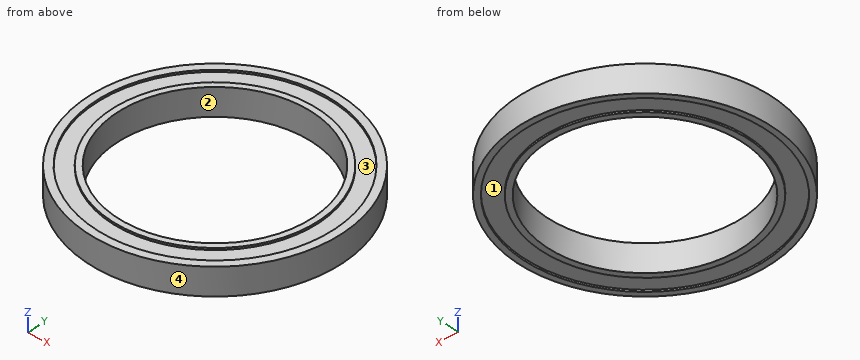
from build123d import *

# Parameters (mm, degrees)
SKETCH010_R     = 32.5
SKETCH010_R_2   = 25
PAD007_DEPTH    = 7
SKETCH011_R     = 30.5
SKETCH011_R_2   = 26.5
POCKET004_DEPTH = 0.5
SKETCH012_R     = 31
SKETCH012_R_2   = 26.5
POCKET005_DEPTH = 0.5


with BuildPart() as part:
    # Sketch010 → Pad007 (new body)
    with BuildSketch(Plane.XY):
        Circle(SKETCH010_R)
        Circle(SKETCH010_R_2, mode=Mode.SUBTRACT)
    extrude(amount=PAD007_DEPTH)

    # Sketch011 → Pocket004 (cut)
    with BuildSketch(Plane.XY.offset(7)):
        Circle(SKETCH011_R)
        Circle(SKETCH011_R_2, mode=Mode.SUBTRACT)
    extrude(amount=-POCKET004_DEPTH, mode=Mode.SUBTRACT)

    # Sketch012 → Pocket005 (cut)
    with BuildSketch(Plane.XY):
        Circle(SKETCH012_R)
        Circle(SKETCH012_R_2, mode=Mode.SUBTRACT)
    extrude(amount=POCKET005_DEPTH, mode=Mode.SUBTRACT)


solid = part.part
Design review of the part built by this model. Coordinates are the model's own, in mm. Face numbers are marked on the shaded views. A direction names the side the tool comes from. Round coordinates to 2 decimals unless told otherwise and drop trailing zeros. Order: outer loops, then holes, each group sorted by start corner. A loop starts at its lowest first (then second) coordinate and runs counter-clockwise, first axis right, second up.
1) Draft analysis for pull direction Y (two halves, no side actions). For the marked faces 3 and 4, state which applies: released by +Y, released by -Y, zero draft, split by the parting line, or undercut.
The answers:
face 3: undercut
face 4: split by the parting line
2) Consider section A-A (y = 0). State the section outline as (x, z) points.
The answers:
outline: (-32.5, 0) - (-31, 0) - (-31, 0.5) - (-26.5, 0.5) - (-26.5, 0) - (-25, 0) - (-25, 7) - (-26.5, 7) - (-26.5, 6.5) - (-30.5, 6.5) - (-30.5, 7) - (-32.5, 7) - close; (25, 0) - (26.5, 0) - (26.5, 0.5) - (31, 0.5) - (31, 0) - (32.5, 0) - (32.5, 7) - (30.5, 7) - (30.5, 6.5) - (26.5, 6.5) - (26.5, 7) - (25, 7) - close
3) Clearance check with flat-ended pins moving along their axes: pin 1 Ø2 at (y, z) = (24, 3) entering from +X; pin 2 Ø2 at (y, z) = (-25, 3.5) entering from -X; pin 3 Ø1.5 at (x, y) = (-21, -24.5) entering from -Z; pin 4 Ø2 at (x, y) = (-20, -11) entering from +Z. State where each tip first meets the part, or that it passes through.
The answers:
pin 1: stops at x = 22.96
pin 2: stops at x = -21.91
pin 3: stops at z = 0
pin 4: passes through
4) Consider section C-C (z = 2.25). State the section outline as (x, y) points.
The answers:
outline: circle Ø65 at (0, 0); hole circle Ø50 at (0, 0)
5) For L1, parallel to Y at x = 0, z = 6.85; L2, parallel to Y at x = 0, z = 0.45; L3, parallel to Y at x = 0, z = 3, list the stretches that pass through material, from the lowest coordinate up.
The answers:
L1: y = -32.5 to -30.5, -26.5 to -25, 25 to 26.5, 30.5 to 32.5
L2: y = -32.5 to -31, -26.5 to -25, 25 to 26.5, 31 to 32.5
L3: y = -32.5 to -25, 25 to 32.5
6) Machinability: for the marked faces 1 and 2, which of the approach directions +Z, -Z, +X, -X, +Y, -Y give a long, thin tool a straight path to every point of the face, cutting with its end or side? Answer none if there is none.
The answers:
face 1: -Z
face 2: +Z, -Z
